Design review of the part shown in the three views and the two pictorial views. Dimensions are in mm from the part's minimum x, y and z. A direction names the side the tool comes from. Coordinates: 2 decimals unless noted, no trailing zeros. Write each loop counter-clockwise with the first axis right and the second up, starting at its lowest first coordinate (ties: lowest second). Pieces come first, ordered by that corner, then holes. Notation, with made-up numbers: (27.5, 81.25) -> (46.5, 81.25) arc R23 cw to (46.5, 96.25) -> close; hole circle Ø11 at (12, -9.75). An arc over 180 degrees is marked (long way). Write each question's results on one line, items separated by ' | '.
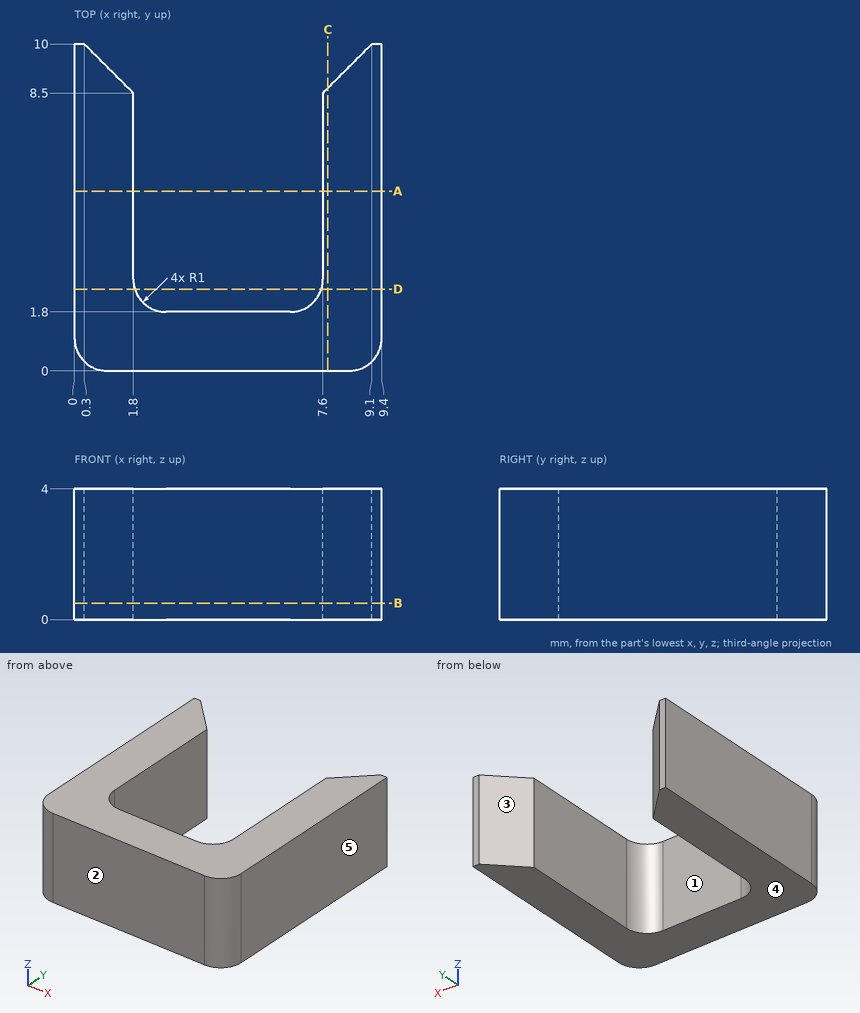
Q1. Add section C-C (x = 7.75). Write out the cut boundary in (y, z).
Solution:
outline: (0, 0) -> (8.65, 0) -> (8.65, 4) -> (0, 4) -> close
Q2. Draft analysis for pull direction X (two halves, no side actions). For the marked faces 3, 4 and 5, state which applies: pulls with the +X half, pulls with the -X half, needs draft (parallel to the pull), parting line crosses it, or undercut.
Solution:
face 3: undercut | face 4: needs draft | face 5: pulls with the +X half
Q3. For line 1 (X direction, y = 8.25, z = 1); line 2 (Y direction, x = 5.25, z = 2.4); line 3 (X direction, y = 9, z = 3), list the stretches that pass through material, from the lowest coordinate up. Write a range as from..to.
Solution:
line 1: 0..1.8, 7.6..9.4 | line 2: 0..1.8 | line 3: 0..1.3, 8.1..9.4
Q4. Clearance check with flat-ended pins moving along their axes: P1, Ø1.5, axis at x = 6, y = 7, coming from the +Z side; P2, Ø1.5, axis at x = 3, z = 2, coming from the +Y side. State where each tip first meets the part, or that it passes through.
Solution:
P1: through | P2: y = 1.96
Q5. Add section D-D (y = 2.5). Write out the cut boundary in (x, z), plus the area to 3 significant figures.
Solution:
outline: (0, 0) -> (1.85, 0) -> (1.85, 4) -> (0, 4) -> close; (7.55, 0) -> (9.4, 0) -> (9.4, 4) -> (7.55, 4) -> close | area: 14.8 mm²
Q6. Add section B-B (z = 0.5). Write out the cut boundary in (x, y).
Solution:
outline: (0, 1) arc R1 ccw to (1, 0) -> (8.4, 0) arc R1 ccw to (9.4, 1) -> (9.4, 10) -> (9.1, 10) -> (7.6, 8.5) -> (7.6, 2.8) arc R1 cw to (6.6, 1.8) -> (2.8, 1.8) arc R1 cw to (1.8, 2.8) -> (1.8, 8.5) -> (0.3, 10) -> (0, 10) -> close
Q7. Machinability: for the marked faces 1 and 2, which of the approach directions +Z, -Z, +X, -X, +Y, -Y give a long, thin tool a straight path to every point of the face, cutting with its end or side? Answer none if there is none.
Solution:
face 1: +Z, -Z, +Y | face 2: +Z, -Z, +X, -X, -Y
Q8. Add section A-A (y = 5.5). Write out the cut boundary in (x, z).
Solution:
outline: (0, 0) -> (1.8, 0) -> (1.8, 4) -> (0, 4) -> close; (7.6, 0) -> (9.4, 0) -> (9.4, 4) -> (7.6, 4) -> close
